from build123d import *

# Parameters (mm, degrees)
SKETCH1_W                 = 170
SKETCH1_H                 = 55
BOSS_EXTRUDE1_DEPTH       = 6.35
FILLET1_R                 = 10
F_6_0MM_DOWEL_HOLE1_D     = 6
F_4_0MM_DOWEL_HOLE1_D     = 4
F_4_0MM_DOWEL_HOLE1_DEPTH = 6.35
F_5_0MM_DOWEL_HOLE1_D     = 5


with BuildPart() as part:
    # Sketch1 → Boss-Extrude1 (new body)
    with BuildSketch(Plane(origin=(0, 0, 0), x_dir=(1, 0, 0), z_dir=(0, 1, 0))):
        with Locations((60, 0)):
            Rectangle(SKETCH1_W, SKETCH1_H)
    extrude(amount=BOSS_EXTRUDE1_DEPTH)

    # Fillet1
    fillet1_edges = [part.edges().sort_by_distance(p)[0] for p in [
        (-25, 3.175, -27.5),
        (145, 3.175, -27.5),
        (145, 3.175, 27.5),
        (-25, 3.175, 27.5),
    ]]
    fillet(fillet1_edges, radius=FILLET1_R)

    # Ø6.0mm Dowel Hole1 (through all)
    with Locations(Plane(origin=(0, 6.35, 0), x_dir=(1, 0, 0), z_dir=(0, 1, 0))):
        with Locations((0, 0)):
            Hole(F_6_0MM_DOWEL_HOLE1_D / 2)

    # Ø4.0mm Dowel Hole1
    with Locations(Plane(origin=(0, 6.35, 0), x_dir=(1, 0, 0), z_dir=(0, 1, 0))):
        with Locations((-16.25, -18.75), (20, -18.75), (95, -18.75), (170, -18.75), (170, 18.75), (95, 18.75), (20, 18.75), (-16.25, 18.75)):
            Hole(F_4_0MM_DOWEL_HOLE1_D / 2, depth=F_4_0MM_DOWEL_HOLE1_DEPTH)

    # Ø5.0mm Dowel Hole1 (through all)
    with Locations(Plane(origin=(0, 6.35, 0), x_dir=(1, 0, 0), z_dir=(0, 1, 0))):
        with Locations((140, 20.5), (120, 20.5), (140, -20.5), (120, -20.5)):
            Hole(F_5_0MM_DOWEL_HOLE1_D / 2)


solid = part.part
CAD build for the part. Positions are in the model's coordinates, mm. Coordinates: 2 decimals unless noted, no trailing zeros. Write each loop counter-clockwise with the first axis right and the second up, starting at its lowest first coordinate (ties: lowest second). Pieces come first, ordered by that corner, then holes. Notation, with made-up numbers: M -35,89 L 19,89 A9 cw 19,94 Z; hole C 87.25,33.25 d8. An arc over 180 degrees is marked long. Answer as a JSON object with one key per item and string values. Group by question number.
1) Saw through at B-B (y = 1.5). Give the number of separate pieces and of enclosed holes in the cut face, plus the area to 3 significant figures.
2) Saw through at C-C (x = 140). Write the cut outline in (y, z).
3) Pin check, flat tip, straight feed: pin 1 Ø3 at (x, z) = (140, 20.5) entering from -Y. Stop position of the tip, or through.
4) Saw through at A-A (x = 95). Write the cut outline in (y, z), plus the area to 3 significant figures.
5) Wall check: line 1 (Z direction, x = 120, y = 4); line 2 (Z direction, x = 95, y = 2); line 3 (X direction, y = 2, z = 20.5). Give the ranges that are in metal, low to high. Write a range as from..to.
6) Mould opens along X. For faces 1 (the face through (59, 6.35, 0)), 2 (the face through (141.99, 3.22, 24.65)), 3 (the face through (20.26, 3.131, -20.733)) say: +X half, -X half, draft (parallel to the pull), parting line (faces both ways), or undercut.
Values follow:
{
 "1": {"separate pieces": "1", "enclosed holes": "11", "area": "9,080 mm2"},
 "2": {"outline": "M 0,-26.16 L 6.35,-26.16 L 6.35,-23 L 0,-23 Z; M 0,-18 L 6.35,-18 L 6.35,18 L 0,18 Z; M 0,23 L 6.35,23 L 6.35,26.16 L 0,26.16 Z"},
 "3": {"pin 1": "passes through"},
 "4": {"outline": "M 0,-27.5 L 6.35,-27.5 L 6.35,-20.75 L 0,-20.75 Z; M 0,-16.75 L 6.35,-16.75 L 6.35,16.75 L 0,16.75 Z; M 0,20.75 L 6.35,20.75 L 6.35,27.5 L 0,27.5 Z", "area": "298 mm2"},
 "5": {"line 1": "z = -27.5..-23, -18..18, 23..27.5", "line 2": "z = -27.5..-20.75, -16.75..16.75, 20.75..27.5", "line 3": "x = -24.54..-17.22, -15.28..19.03, 20.97..94.03, 95.97..117.5, 122.5..137.5, 142.5..144.54"},
 "6": {"face 1": "draft", "face 2": "+X half", "face 3": "undercut"}
}
